from build123d import *

# Parameters (mm, degrees)
F0_W      = 15
F0_H      = 15
F1_DEPTH  = 7.5
F2_DEPTH  = 2
F3_W      = 5.1
F3_H      = 5.1
F4_DEPTH  = 25
F5_DEPTH  = 2
F6_W      = 19
F6_H      = 19
F7_DEPTH  = 10
F8_R      = 5
F9_R      = 5.9
F9_R_2    = 3.9
F10_DEPTH = 2
F11_DEPTH = 25


with BuildPart() as f1:
    # F0 (on Top) → F1 (new body)
    with BuildSketch(Plane.XY):
        Rectangle(F0_W, F0_H)
        with BuildLine():
            ThreePointArc((3.7416573868, 1.1), (3.8602113808, 0.5556690524), (3.9, 0))
            ThreePointArc((3.9, 0), (3.8602113808, -0.5556690524), (3.7416573868, -1.1))
            ThreePointArc((3.7416573868, -1.1), (0, -3.9), (-3.7416573868, -1.1))
            ThreePointArc((-3.7416573868, -1.1), (-3.9, 0), (-3.7416573868, 1.1))
            ThreePointArc((-3.7416573868, 1.1), (0, 3.9), (3.7416573868, 1.1))
        make_face(mode=Mode.SUBTRACT)
        with BuildLine():
            ThreePointArc((-3.7416573868, -1.1), (0, -3.9), (3.7416573868, -1.1))
            Line((3.7416573868, -1.1), (-3.7416573868, -1.1))
        make_face()
        with BuildLine():
            Line((-3.7416573868, 1.1), (3.7416573868, 1.1))
            ThreePointArc((3.7416573868, 1.1), (0, 3.9), (-3.7416573868, 1.1))
        make_face()
        with BuildLine():
            ThreePointArc((3.7416573868, -1.1), (3.8602113808, -0.5556690524), (3.9, 0))
            ThreePointArc((3.9, 0), (3.8602113808, 0.5556690524), (3.7416573868, 1.1))
            Line((3.7416573868, 1.1), (-3.7416573868, 1.1))
            ThreePointArc((-3.7416573868, 1.1), (-3.9, 0), (-3.7416573868, -1.1))
            Line((-3.7416573868, -1.1), (3.7416573868, -1.1))
        make_face()
    extrude(amount=F1_DEPTH)

    # F0 (on Top) → F2 (join)
    with BuildSketch(Plane.XY):
        with BuildLine():
            ThreePointArc((3.7416573868, -1.1), (3.8602113808, -0.5556690524), (3.9, 0))
            ThreePointArc((3.9, 0), (3.8602113808, 0.5556690524), (3.7416573868, 1.1))
            Line((3.7416573868, 1.1), (-3.7416573868, 1.1))
            ThreePointArc((-3.7416573868, 1.1), (-3.9, 0), (-3.7416573868, -1.1))
            Line((-3.7416573868, -1.1), (3.7416573868, -1.1))
        make_face()
    extrude(amount=F2_DEPTH)

    # F3 (on face) → F4 (join)
    with BuildSketch(Plane(origin=(0, 0, 0), x_dir=(1, 0, 0), z_dir=(0, 0, -1))):
        with Locations((-4.95, -4.95)):
            Rectangle(F3_W, F3_H)
        with Locations((4.95, -4.95)):
            Rectangle(F3_W, F3_H)
        with Locations((4.95, 4.95)):
            Rectangle(F3_W, F3_H)
        with Locations((-4.95, 4.95)):
            Rectangle(F3_W, F3_H)
    extrude(amount=F4_DEPTH)

    # F5 (add): a face of the model
    f5_faces = [f1.faces().sort_by_distance(p)[0] for p in [
        (0, 0, 7.5),
    ]]
    extrude(f5_faces, amount=F5_DEPTH)

    # F6 (on face) → F7 (join)
    with BuildSketch(Plane(origin=(0, 0, -25), x_dir=(1, 0, 0), z_dir=(0, 0, -1))):
        Rectangle(F6_W, F6_H)
        Polygon((-7.5, 2.4), (-7.5, 7.5), (-2.4, 7.5), (2.4, 7.5), (7.5, 7.5), (7.5, 2.4), (7.5, -2.4), (7.5, -7.5), (2.4, -7.5), (-2.4, -7.5), (-7.5, -7.5), (-7.5, -2.4), align=None, mode=Mode.SUBTRACT)
    extrude(amount=-F7_DEPTH)

    # F8
    f8_edges = [f1.edges().sort_by_distance(p)[0] for p in [
        (9.5, -9.5, -20),
        (9.5, 9.5, -20),
        (-9.5, 9.5, -20),
        (-9.5, -9.5, -20),
    ]]
    fillet(f8_edges, radius=F8_R)

    # F9 (on face) → F10 (join)
    with BuildSketch(Plane.XY.offset(9.5)):
        Circle(F9_R)
        Circle(F9_R_2, mode=Mode.SUBTRACT)
    extrude(amount=F10_DEPTH)

    # F11 (add): a face of the model
    f11_faces = [f1.faces().sort_by_distance(p)[0] for p in [
        (0, 0, 9.5),
    ]]
    extrude(f11_faces, amount=F11_DEPTH)


solid = f1.part
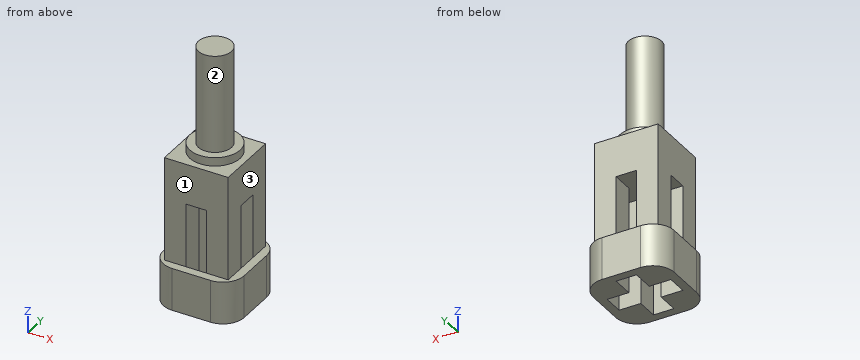
Design review of the part built by this model. Coordinates are the model's own, in mm. Face numbers are marked on the shaded views. A direction names the side the tool comes from. Coordinates: 2 decimals unless noted, no trailing zeros. Order: outer loops, then holes, each group sorted by start corner. A loop starts at its lowest first (then second) coordinate and runs counter-clockwise, first axis right, second up. Notation, with made-up numbers: (-2.75, 14) -> (51.25, 14) arc R29 cw to (51.25, 46) -> close; hole circle Ø5 at (33, 30). An arc over 180 degrees is marked (long way). Use one line per item in the form item = value. Start each with the question number.
(1) Insertion check: pin 1 (5.5 mm diameter, centred on y = 6, z = -9.5, fed in from -X); pin 2 (4 mm diameter, centred on x = 5.5, z = 7.5, fed in from -Y); pin 3 (1.5 mm diameter, centred on y = -5.5, z = -15.5, fed in from -X); pin 4 (6 mm diameter, centred on x = 2, y = 3.5, fed in from -Z). Each pin has a flat end and moves straight along its axis. Give the tip position at first contact, or say it passes through.
(2) For the marked faces 1, 2 and 3, list the 3-axis set-ups (+Z, -Z, +X, -X, +Y, -Y) from which the entire face can be reached by the end or side of a thin tool; tool diameter is ignored.
(3) Add section A-A on x = 0. State the section outline as (y, z) points.
(4) Add section D-D on z = 17.5. State the section outline as (x, y) points.
(5) For probe 1 along Y at (x, z) = (1.25, -15.5); probe 2 along Y at (x, z) = (3.75, -11), list the stretches that pass through material, from the lowest coordinate up.
(6) Add section B-B on z = -2. State the section outline as (x, y) points, plus the area to 3 significant figures.
Answer block:
q1.pin_1 = -7.5
q1.pin_2 = -7.5
q1.pin_3 = -9.49
q1.pin_4 = -25
q2.face_1 = +Z, +X, -X, -Y
q2.face_2 = +Z
q2.face_3 = +Z, +X, +Y, -Y
q3.outline = (-9.5, -25) -> (-7.5, -25) -> (-7.5, -15) -> (-9.5, -15) -> close; (-7.5, 0) -> (7.5, 0) -> (7.5, 9.5) -> (5.9, 9.5) -> (5.9, 11.5) -> (3.9, 11.5) -> (3.9, 34.5) -> (-3.9, 34.5) -> (-3.9, 11.5) -> (-5.9, 11.5) -> (-5.9, 9.5) -> (-7.5, 9.5) -> close; (7.5, -25) -> (9.5, -25) -> (9.5, -15) -> (7.5, -15) -> close
q4.outline = circle Ø7.8 at (0, 0)
q5.probe_1 = -9.5 to -7.5, 7.5 to 9.5
q5.probe_2 = -7.5 to -2.4, 2.4 to 7.5
q6.outline = (-7.5, -7.5) -> (-2.4, -7.5) -> (-2.4, -2.4) -> (-7.5, -2.4) -> close; (-7.5, 2.4) -> (-2.4, 2.4) -> (-2.4, 7.5) -> (-7.5, 7.5) -> close; (2.4, -7.5) -> (7.5, -7.5) -> (7.5, -2.4) -> (2.4, -2.4) -> close; (2.4, 2.4) -> (7.5, 2.4) -> (7.5, 7.5) -> (2.4, 7.5) -> close
q6.area = 104 mm²
